from build123d import *

# Parameters (mm, degrees)
F1_DEPTH = 29
F2_W     = 124.405438
F2_H     = 36
F3_DEPTH = 11
F5_DEPTH = 38.001


with BuildPart() as f1:
    # F0 (on Front) → F1 (new body, symmetric)
    with BuildSketch(Plane.XZ):
        with BuildLine():
            Line((-52.5, 0), (0, 0))
            Line((0, 0), (52.5, 0))
            Line((52.5, 0), (52.5, 9))
            Line((52.5, 9), (63.5, 9))
            ThreePointArc((63.5, 9), (62.202719, 25.094135), (52.5, 38))
            Line((52.5, 38), (0, 38))
            Line((0, 38), (-52.5, 38))
            ThreePointArc((-52.5, 38), (-62.202719, 25.094135), (-63.5, 9))
            Line((-63.5, 9), (-52.5, 9))
            Line((-52.5, 9), (-52.5, 0))
        make_face()
    extrude(amount=F1_DEPTH, both=True)

    # F2 (on face) → F3 (cut)
    with BuildSketch(Plane.XY.offset(38)):
        Rectangle(F2_W, F2_H)
    extrude(amount=-F3_DEPTH, mode=Mode.SUBTRACT)

    # F4 (on Top) → F5 (cut, through all)
    with BuildSketch(Plane.XY):
        with BuildLine():
            Line((-19.5, 6.5), (-38.5, 6.5))
            ThreePointArc((-38.5, 6.5), (-45, 0), (-38.5, -6.5))
            Line((-38.5, -6.5), (-19.5, -6.5))
            ThreePointArc((-19.5, -6.5), (-13, 0), (-19.5, 6.5))
        make_face()
        with BuildLine():
            ThreePointArc((19.5, 6.5), (13, 0), (19.5, -6.5))
            Line((19.5, -6.5), (38.5, -6.5))
            ThreePointArc((38.5, -6.5), (45, 0), (38.5, 6.5))
            Line((38.5, 6.5), (19.5, 6.5))
        make_face()
    extrude(amount=F5_DEPTH, mode=Mode.SUBTRACT)


solid = f1.part
Geometry check sheet. Reference: the model listing, model coordinates, mm. A direction names the side the tool comes from. Round coordinates to 2 decimals unless told otherwise and drop trailing zeros. Loops run counter-clockwise (first coordinate to the right, second up) from the corner with the lowest first, then second, coordinate; pieces in that order, holes last. Notation, with made-up numbers: (13, 46.5) -> (42, 46.5) arc R28 ccw to (42, 79.5) -> close; hole circle Ø2 at (29.5, -22.5). An arc over 180 degrees is marked (long way). Answer as a JSON object with one key per item and string values. Group by question number.
Item 1: Depth check by flat-ended pin: pin 1 Ø10 at (y, z) = (-10, 29.5) entering from -X; pin 2 Ø3.5 at (x, y) = (-60, -3) entering from -Z; pin 3 Ø12 at (y, z) = (-17.5, 8.5) entering from +X. Enter the tip coordinate at first touch or a pass-through.
Item 2: Set-up check for faces 4 (the face through (52.5, 0, 4)), 5 (the face through (63.33, -0.41, 21.4)), 6 (the face through (-29, 6.5, 13)), 7 (the face through (-1, 0, 27)), 8 (the face through (-52.5, 0, 5)): record each of +Z, -Z, +X, -X, +Y, -Y from which the full face is reachable in a straight line by a thin tool's end or side.
Item 3: Cross-section at A-A, the plane z = 6. Record the cut outline in (x, y).
Item 4: Cross-section at D-D, the plane y = 8.5. Record the cut outline in (x, z).
Item 5: Cross-section at C-C, the plane y = 0. Record the cut outline in (x, z).
Item 6: Thickness scan on line 1 along X through (y, z) = (-0.5, 3); line 2 along Y through (x, z) = (-15.5, 35.5); line 3 along Y through (x, z) = (23.5, 15). Record the ranges inside material, lowest first.
Item 7: Release check for a two-part mould opening along Y. For faces 1 (the face through (-1, 29, 19)), 2 (the face through (-13, 0, 13)), 3 (the face through (1, -24, 38)) record: pulls with the +Y half, pulls with the -Y half, needs draft (parallel to the pull), parting line crosses it, or undercut.
Item 8: Cross-section at B-B, the plane x = 32. Record the cut outline in (y, z).
Determined:
{
 "1": {"pin 1": "stops at x = -62.42", "pin 2": "stops at z = 9", "pin 3": "stops at x = 64.09"},
 "2": {"face 4": "-Z, +X, +Y, -Y", "face 5": "+X, +Y, -Y", "face 6": "+Z, -Z", "face 7": "+Z, +X, -X", "face 8": "-Z, -X, +Y, -Y"},
 "3": {"outline": "(-52.5, -29) -> (52.5, -29) -> (52.5, 29) -> (-52.5, 29) -> close; hole (-38.5, -6.5) -> (-19.5, -6.5) arc R6.5 ccw to (-19.5, 6.5) -> (-38.5, 6.5) arc R6.5 ccw to start; hole (19.5, -6.5) -> (38.5, -6.5) arc R6.5 ccw to (38.5, 6.5) -> (19.5, 6.5) arc R6.5 ccw to start"},
 "4": {"outline": "(-63.5, 9) -> (-52.5, 9) -> (-52.5, 0) -> (52.5, 0) -> (52.5, 9) -> (63.5, 9) arc R29 ccw to (61.4, 27) -> (-61.4, 27) arc R29 ccw to start"},
 "5": {"outline": "(-63.5, 9) -> (-52.5, 9) -> (-52.5, 0) -> (-45, 0) -> (-45, 27) -> (-61.4, 27) arc R29 ccw to start; (-13, 0) -> (13, 0) -> (13, 27) -> (-13, 27) -> close; (45, 0) -> (52.5, 0) -> (52.5, 9) -> (63.5, 9) arc R29 ccw to (61.4, 27) -> (45, 27) -> close"},
 "6": {"line 1": "x = -52.5 to -44.98, -13.02 to 13.02, 44.98 to 52.5", "line 2": "y = -29 to -18, 18 to 29", "line 3": "y = -29 to -6.5, 6.5 to 29"},
 "7": {"face 1": "pulls with the +Y half", "face 2": "undercut", "face 3": "needs draft"},
 "8": {"outline": "(-29, 0) -> (-6.5, 0) -> (-6.5, 27) -> (-18, 27) -> (-18, 38) -> (-29, 38) -> close; (6.5, 0) -> (29, 0) -> (29, 38) -> (18, 38) -> (18, 27) -> (6.5, 27) -> close"}
}
